from build123d import *

# Parameters (mm, degrees)
SKETCH1_R               = 16
BOSS_EXTRUDE1_DEPTH     = 88
SKETCH2_R               = 14.360467733
CUT_EXTRUDE1_DEPTH      = 88
SKETCH3_W               = 41.504964389
SKETCH3_H               = 7.516490838
CUT_EXTRUDE2_DEPTH      = 88
CUT_EXTRUDE3_DEPTH      = 91.862533533
CUT_EXTRUDE3_DEPTH_BACK = 91.862533533


with BuildPart() as part:
    # Sketch1 → Boss-Extrude1 (new body)
    with BuildSketch(Plane.XY):
        Circle(SKETCH1_R)
    extrude(amount=BOSS_EXTRUDE1_DEPTH)

    # Sketch2 → Cut-Extrude1 (cut)
    with BuildSketch(Plane.XY.offset(88)):
        Circle(SKETCH2_R)
    extrude(amount=-CUT_EXTRUDE1_DEPTH, mode=Mode.SUBTRACT)

    # Sketch3 → Cut-Extrude2 (cut)
    with BuildSketch(Plane.XY.offset(88)):
        with Locations((1.087364542, -14.00175825)):
            Rectangle(SKETCH3_W, SKETCH3_H)
    extrude(amount=-CUT_EXTRUDE2_DEPTH, mode=Mode.SUBTRACT)

    # Sketch4 → Cut-Extrude3 (cut, two sides: drawn at the far end of the back side and taken through both)
    with BuildSketch(Plane(origin=(0, 0, 0), x_dir=(0, 0, -1), z_dir=(1, 0, 0)).offset(-CUT_EXTRUDE3_DEPTH_BACK)):
        Polygon((9.063254849, -11.588963216), (-25.804371383, 15.282726161), (-30.207370546, 20.432915897), (5.089153987, 19.311664184), align=None)
    extrude(amount=CUT_EXTRUDE3_DEPTH + CUT_EXTRUDE3_DEPTH_BACK, mode=Mode.SUBTRACT)


solid = part.part
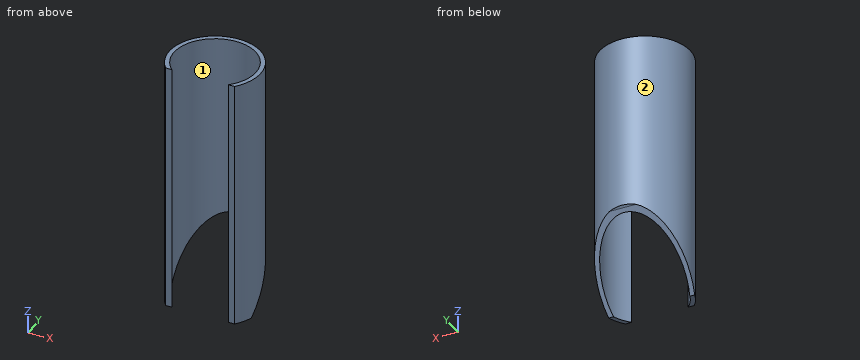
Read the model definition and answer for the solid it produces. Units are mm, in the model's axes. Face numbers are marked on the shaded views. Coordinates: 2 decimals unless noted, no trailing zeros. Order: outer loops, then holes, each group sorted by start corner. A loop starts at its lowest first (then second) coordinate and runs counter-clockwise, first axis right, second up. Notation, with made-up numbers: (3.25, 55.5) - (51.25, 55.5) arc R14 cw to (51.25, 78.5) - close; hole circle Ø2 at (-4, 86). An arc over 180 degrees is marked (long way). Use one line per item in the form item = value.
(1) Section C-C, the plane z = 35.5 is taken. Give the vertices of the cut face in (x, y), then the cut area to 3 significant figures.
Computed values:
outline = (-12.29, -10.24) - (-10.06, -10.24) arc R14.36 cw (long way) to (10.06, -10.24) - (12.29, -10.24) arc R16 ccw (long way) to start
area = 115 mm²
(2) Straight lines are drawn through the part: L1, parallel to X at y = 0, z = 56; L2, parallel to Y at x = 0, z = 33; L3, parallel to X at y = -6.5, z = 27.5. For each, find the intervals that lie inside material, in ascending order.
Computed values:
L1 = -16 to -14.36, 14.36 to 16
L2 = 14.36 to 16
L3 = -14.62 to -12.81, 12.81 to 14.62
(3) For a pull along Y with two mould halves and no side action, classify the marked faces 1 and 2 as pulls with the +Y half, pulls with the -Y half, needs draft (parallel to the pull), parting line crosses it, or undercut.
Computed values:
face_1 = undercut
face_2 = parting line crosses it
(4) Given pin 1 Ø5 at (x, z) = (-10, 37.5) entering from +Y, flat-ended and moving along its own axis, determine where the tip first touches the part or whether it passes through.
Computed values:
pin_1 = 14.13
(5) Section D-D, the plane y = 12.5 is taken. Give the vertices of the cut face in (x, z), then the cut area to 3 significant figures.
Computed values:
outline = (-9.99, 22.19) - (-7.07, 22.19) - (-7.07, 88) - (-9.99, 88) - close; (7.07, 22.19) - (9.99, 22.19) - (9.99, 88) - (7.07, 88) - close
area = 384 mm²
(6) Section A-A, the plane y = 0 is taken. Give the vertices of the cut face in (x, z).
Computed values:
outline = (-16, 5.97) - (-14.36, 5.97) - (-14.36, 88) - (-16, 88) - close; (14.36, 5.97) - (16, 5.97) - (16, 88) - (14.36, 88) - close
(7) Section B-B, the plane x = 0 is taken. Give the vertices of the cut face in (y, z), then the cut area to 3 significant figures.
Computed values:
outline = (14.36, 24.61) - (15.28, 25.8) - (16, 26.42) - (16, 88) - (14.36, 88) - close
area = 102 mm²
